from build123d import *

# Parameters (mm, degrees)
SKETCH2_R           = 6.35
BOSS_EXTRUDE1_DEPTH = 9.525
SKETCH4_R           = 6.35
BOSS_EXTRUDE3_DEPTH = 25.4


with BuildPart() as part:
    # Sketch2 → Boss-Extrude1 (new body)
    with BuildSketch(Plane(origin=(0, 0, 0), x_dir=(0, 0, -1), z_dir=(1, 0, 0))):
        with BuildLine():
            Line((0, 12.7), (381, 12.7))
            ThreePointArc((381, 12.7), (393.7, 0), (381, -12.7))
            Line((381, -12.7), (0, -12.7))
            ThreePointArc((0, -12.7), (-12.7, 0), (0, 12.7))
        make_face()
        with Locations(Location((0, 0, 0), (0, 0, 180))):
            Circle(SKETCH2_R, mode=Mode.SUBTRACT)
    extrude(amount=BOSS_EXTRUDE1_DEPTH)

    # Sketch4 → Boss-Extrude3 (add)
    with BuildSketch(Plane.ZY):
        with Locations(Location((-381, 0, 0), (0, 0, 180))):
            Circle(SKETCH4_R)
    extrude(amount=BOSS_EXTRUDE3_DEPTH)


solid = part.part
Work out the finished part from the listing and answer in its coordinate system (mm). A direction names the side the tool comes from. Give positions to 0.01 mm unless a question says otherwise; leave off trailing zeros. Write each loop counter-clockwise with the first axis right and the second up, starting at its lowest first coordinate (ties: lowest second). Pieces come first, ordered by that corner, then holes.
Q1. A tool of negligible diameter and unlimited length cuts with its end or side. For faces 1 (the face through (5, 12.7, -188)), 2 (the face through (-12.522, -0.279, -374.656)), from which of +Z, -Z, +X, -X, +Y, -Y can it reach the whole face along a straight path? Write none if from no direction.
Answer:
face 1: +Z, -Z, +X, -X, +Y
face 2: -X
Q2. For a pull along Y with two mould halves and no side action, classify faces 3 (the face through (-25.4, 0, -381)), 4 (the face through (4.696, 5.634, 2.93)), 5 (the face through (5, -12.7, -193)) as released by +Y, released by -Y, zero draft, split by the parting line, or undercut.
Answer:
face 3: zero draft
face 4: undercut
face 5: released by -Y
Q3. The part is cut by section B-B on x = 6. Give the vertices of the cut face in (y, z), and give its area (3 significant figures).
Answer:
outline: (-12.7, -381) arc R12.7 ccw to (12.7, -381) - (12.7, 0) arc R12.7 ccw to (-12.7, 0) - close; hole circle Ø12.7 at (0, 0)
area: 10,100 mm2
Q4. The part is cut by section D-D on x = -14.5. Give the vertices of the cut face in (y, z), and give its area (3 significant figures).
Answer:
outline: circle Ø12.7 at (0, -381)
area: 127 mm2
Q5. Given pin 1 (5 mm diameter, centred on y = 6, z = -220, fed in from -X); pin 2 (5 mm diameter, centred on x = -2, y = 2.5, fed in from +Z), each flat-ended and moving along its own axis, determine where each tip first touches the part or whether it passes through.
Answer:
pin 1: stops at x = 0
pin 2: stops at z = 12.66
Q6. Straight lines are drawn through the part: L1, parallel to X at y = -10.25, z = -89.5 (3 decimals); L2, parallel to Z at x = 3, y = 4.25; L3, parallel to Z at x = 6, y = 2. For each, find the intervals that lie inside material, in ascending order.
Answer:
L1: x = 0 to 9.525
L2: z = -392.97 to -4.72, 4.72 to 11.97
L3: z = -393.54 to -6.03, 6.03 to 12.54
Q7. The part is cut by section C-C on z = -169.5. Give the vertices of the cut face in (x, y) (3 decimals).
Answer:
outline: (0, -12.7) - (9.525, -12.7) - (9.525, 12.7) - (0, 12.7) - close
Q8. The part is cut by section A-A on y = 0. Give the vertices of the cut face in (x, z) (3 decimals).
Answer:
outline: (-25.4, -387.35) - (0, -387.35) - (0, -393.7) - (9.525, -393.7) - (9.525, -6.35) - (0, -6.35) - (0, -374.65) - (-25.4, -374.65) - close; (0, 6.35) - (9.525, 6.35) - (9.525, 12.7) - (0, 12.7) - close
